Source: CAD feature listing. Evaluate the final solid. Frame: model axes, mm. Face numbers are marked on the shaded views. A direction names the side the tool comes from. Round coordinates to 2 decimals unless told otherwise and drop trailing zeros. Write each loop counter-clockwise with the first axis right and the second up, starting at its lowest first coordinate (ties: lowest second). Pieces come first, ordered by that corner, then holes. Notation, with made-up numbers: M -16.75,-0.5 L 0.25,-0.5 A33 cw 0.25,28.5 Z; hole C 15,-39.75 d4. An arc over 180 degrees is marked long. Answer in a Markdown table with one row per item. Add a question column.
Item 1: Mould query, pull axis Y, two halves, no side actions, for the marked faces 3, 4 and 5. Classes: released by +Y, released by -Y, zero draft, split by the parting line, or undercut.
Item 2: Cut plane B-B on z = 18. Return loops of the section in (x, y), and give its area (3 significant figures).
Item 3: Cut plane A-A on y = 8. Return loops of the section in (x, z), and give its area (3 significant figures).
Item 4: Contact query for flat-ended pins moving along their axis: pin 1 (1 mm diameter, centred on x = -11.5, z = 38, fed in from -Y); pin 2 (10 mm diameter, centred on y = 0, z = 41.5, fed in from -X). Output: stop coordinate, or through.
Item 5: Set-up query: the marked faces 1 and 2. Return all of +Z, -Z, +X, -X, +Y, -Y with unobstructed straight access to the full face (end or side cutting, diameter ignored); none if empty.
Item 6: Cut plane C-C on x = 4. Return loops of the section in (y, z).
Item 7: Material intervals for probe 1 along X at (y, z) = (7.5, 20.5); probe 2 along Y at (x, z) = (-0.5, 23); probe 3 along X at (y, z) = (18, 18), sorted ascending.
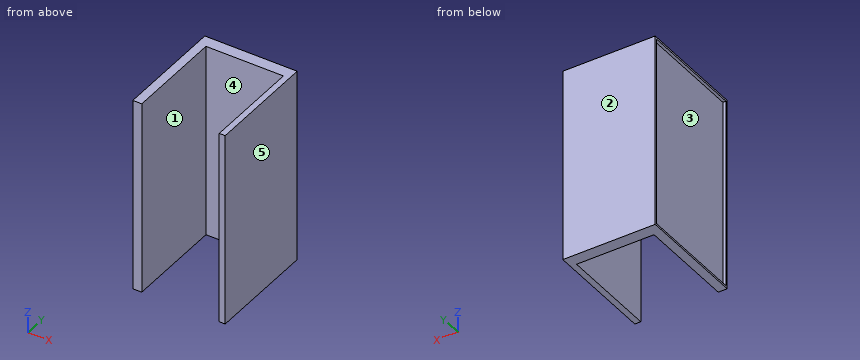
from build123d import *

# Parameters (mm, degrees)
FRONT_PROFILE_DEPTH  = 65.2
SKETCH3_W            = 65.2
SKETCH3_H            = 37
SKETCH3_W_2          = 63.86
SKETCH3_H_2          = 35.66
HOUSING_SNAPON_DEPTH = 1


with BuildPart() as part:
    # Sketch2 → Front Profile (new body)
    with BuildSketch(Plane.XY):
        Polygon((-13, -16.5), (-15, -16.5), (-15, 20.5), (15, 20.5), (15, -16.5), (13, -16.5), (13, 16.5), (-13, 16.5), align=None)
    extrude(amount=FRONT_PROFILE_DEPTH)

    # Sketch3 → Housing SnapOn (add)
    with BuildSketch(Plane.ZY.offset(15)):
        with Locations((32.6, 2)):
            Rectangle(SKETCH3_W, SKETCH3_H)
        with Locations((32.6, 2)):
            Rectangle(SKETCH3_W_2, SKETCH3_H_2, mode=Mode.SUBTRACT)
    extrude(amount=HOUSING_SNAPON_DEPTH)


solid = part.part
Results below:
| question | item | result |
|---|---|---|
| 1 | face 3 | undercut |
| 1 | face 4 | released by -Y |
| 1 | face 5 | zero draft |
| 2 | outline | M -16,-16.5 L -13,-16.5 L -13,16.5 L 13,16.5 L 13,-16.5 L 15,-16.5 L 15,20.5 L -16,20.5 L -16,19.83 L -15,19.83 L -15,-15.83 L -16,-15.83 Z |
| 2 | area | 253 mm2 |
| 3 | outline | M -16,0 L -13,0 L -13,65.2 L -16,65.2 L -16,64.53 L -15,64.53 L -15,0.67 L -16,0.67 Z; M 13,0 L 15,0 L 15,65.2 L 13,65.2 Z |
| 3 | area | 262 mm2 |
| 4 | pin 1 | y = 16.5 |
| 4 | pin 2 | x = -15 |
| 5 | face 1 | +Z, -Z, -Y |
| 5 | face 2 | +Z, -Z, +X, -X, +Y |
| 6 | outline | M 16.5,0 L 20.5,0 L 20.5,65.2 L 16.5,65.2 Z |
| 7 | probe 1 | -15 to -13, 13 to 15 |
| 7 | probe 2 | 16.5 to 20.5 |
| 7 | probe 3 | -15 to 15 |
